Could you check a few things on this drawing? It's one solid part, dimensions in mm from its lowest x, y, z. A direction names the side the tool comes from. Round coordinates to 2 decimals unless told otherwise and drop trailing zeros. Loops run counter-clockwise (first coordinate to the right, second up) from the corner with the lowest first, then second, coordinate; pieces in that order, holes last. Notation, with made-up numbers: (59, -22) -> (72, -22) arc R37 cw to (72, 16) -> close; hole circle Ø10 at (7.25, 15). An arc over 180 degrees is marked (long way). Use one line per item in the form item = value. Start each with the question number.
Item 1: Thinking about a two-plate mould opening in Y: for the marked faces 1, 2 and 3, which applies, released by +Y, released by -Y, zero draft, split by the parting line, or undercut?
Item 2: If we section it at A-A (y = 5): Write out the boundary of the cut face in (x, z).
Item 3: I'm going to push flat-ended pins straight in: pin 1 Ø2 at (x, y) = (5.5, 40.5) entering from -Z; pin 2 Ø2.5 at (y, z) = (21, 3.5) entering from -X. Where does each tip first touch, or does it pass through?
Item 4: If we section it at B-B (x = 5): Write out the boundary of the cut face in (y, z).
Item 5: For the marked faces 4 and 5, which set-ups out of +Z, -Z, +X, -X, +Y, -Y let a thin tool reach every point of the face, with its end or its side?
Item 6: If we section it at D-D (x = 10.5): Write out the boundary of the cut face in (y, z).
Item 7: If I drill on L1, parallel to Y at x = 10.35, z = 4; L2, parallel to Y at x = 5, z = 11.25; L3, parallel to Z at x = 10.85, y = 25, over which ranges is the centre line in solid material (lowest first)? Write a range as [from, to].
Item 8: If we section it at C-C (z = 4): Write out the boundary of the cut face in (x, y).
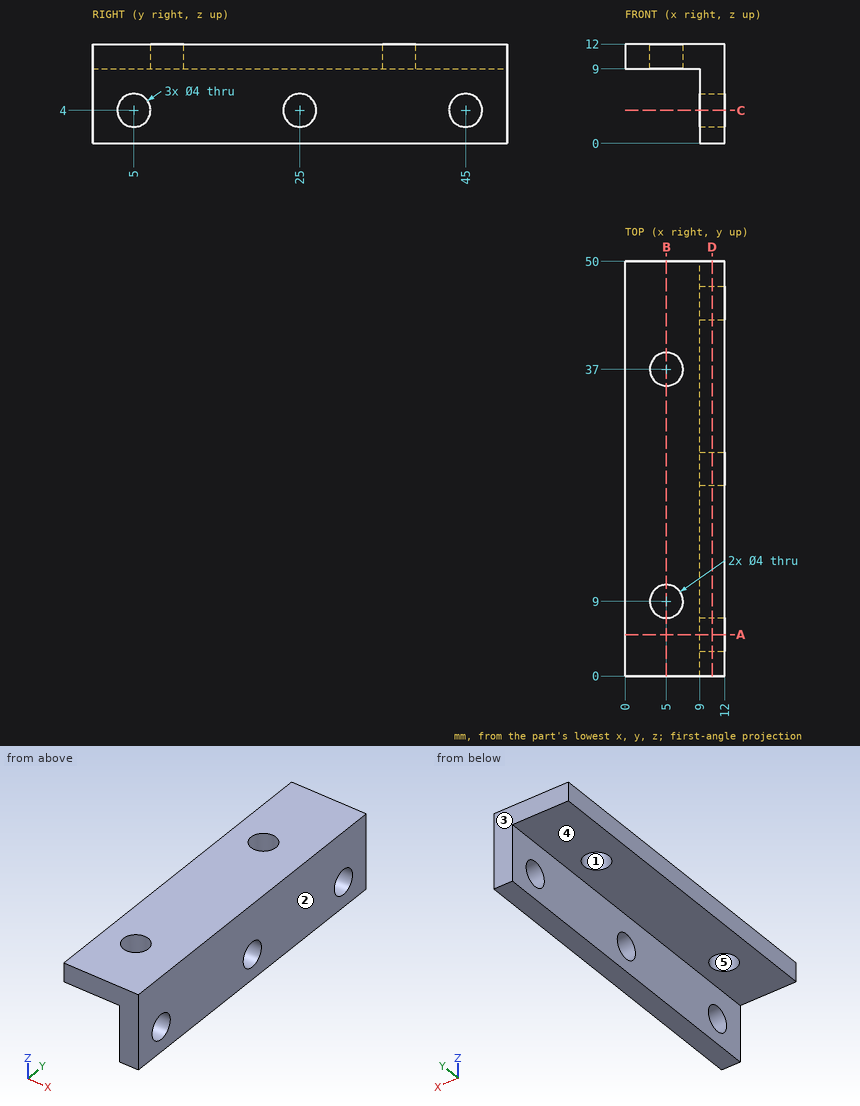
Values found:
q1.face_1 = undercut
q1.face_2 = zero draft
q1.face_3 = released by +Y
q2.outline = (0, 9) -> (9, 9) -> (9, 6) -> (12, 6) -> (12, 12) -> (0, 12) -> close; (9, 0) -> (12, 0) -> (12, 2) -> (9, 2) -> close
q3.pin_1 = 9
q3.pin_2 = 9
q4.outline = (0, 9) -> (7, 9) -> (7, 12) -> (0, 12) -> close; (11, 9) -> (35, 9) -> (35, 12) -> (11, 12) -> close; (39, 9) -> (50, 9) -> (50, 12) -> (39, 12) -> close
q5.face_4 = -Z, -X, +Y, -Y
q5.face_5 = +Z, -Z
q6.outline = (0, 0) -> (50, 0) -> (50, 12) -> (0, 12) -> close; hole circle Ø4 at (5, 4); hole circle Ø4 at (25, 4); hole circle Ø4 at (45, 4)
q7.L1 = [0, 3], [7, 23], [27, 43], [47, 50]
q7.L2 = [0, 7], [11, 35], [39, 50]
q7.L3 = [0, 2], [6, 12]
q8.outline = (9, 0) -> (12, 0) -> (12, 3) -> (9, 3) -> close; (9, 7) -> (12, 7) -> (12, 23) -> (9, 23) -> close; (9, 27) -> (12, 27) -> (12, 43) -> (9, 43) -> close; (9, 47) -> (12, 47) -> (12, 50) -> (9, 50) -> close
